Part model, mm, in its own coordinate system. Round coordinates to 2 decimals unless told otherwise and drop trailing zeros. Return JSON: item names as keys, results as strings. Group by question number.
```python
from build123d import *

# Parameters (mm, degrees)
SKETCH1_R           = 2.1
BOSS_EXTRUDE2_DEPTH = 304.8


with BuildPart() as part:
    # Sketch1 → Boss-Extrude2 (new body)
    with BuildSketch(Plane.XY):
        with BuildLine():
            Line((-8.5, 10), (-4.862792737, 10))
            ThreePointArc((-4.862792737, 10), (-4.598292737, 9.947387679), (-4.374060464, 9.797560464))
            Line((-4.374060464, 9.797560464), (-3.3865, 8.81))
            Line((-3.3865, 8.81), (-3.3865, 8.2))
            Line((-3.3865, 8.2), (-5.5, 8.2))
            Line((-5.5, 8.2), (-5.5, 6.561))
            Line((-5.5, 6.561), (-2.8395, 3.9005))
            Line((-2.8395, 3.9005), (-0.1, 3.9005))
            Line((-0.1, 3.9005), (0, 3.8005))
            Line((0, 3.8005), (0.1, 3.9005))
            Line((0.1, 3.9005), (2.8395, 3.9005))
            Line((2.8395, 3.9005), (5.5, 6.561))
            Line((5.5, 6.561), (5.5, 8.2))
            Line((5.5, 8.2), (3.3865, 8.2))
            Line((3.3865, 8.2), (3.3865, 8.81))
            Line((3.3865, 8.81), (4.374060464, 9.797560464))
            ThreePointArc((4.374060464, 9.797560464), (4.598292737, 9.947387679), (4.862792737, 10))
            Line((4.862792737, 10), (8.5, 10))
            ThreePointArc((8.5, 10), (9.560660172, 9.560660172), (10, 8.5))
            Line((10, 8.5), (10, 4.862792737))
            ThreePointArc((10, 4.862792737), (9.947387679, 4.598292737), (9.797560464, 4.374060464))
            Line((9.797560464, 4.374060464), (8.81, 3.3865))
            Line((8.81, 3.3865), (8.2, 3.3865))
            Line((8.2, 3.3865), (8.2, 5.5))
            Line((8.2, 5.5), (6.561, 5.5))
            Line((6.561, 5.5), (3.9005, 2.8395))
            Line((3.9005, 2.8395), (3.9005, 0.1))
            Line((3.9005, 0.1), (3.8005, 0))
            Line((3.8005, 0), (3.9005, -0.1))
            Line((3.9005, -0.1), (3.9005, -2.8395))
            Line((3.9005, -2.8395), (6.561, -5.5))
            Line((6.561, -5.5), (8.2, -5.5))
            Line((8.2, -5.5), (8.2, -3.3865))
            Line((8.2, -3.3865), (8.81, -3.3865))
            Line((8.81, -3.3865), (9.797560464, -4.374060464))
            ThreePointArc((9.797560464, -4.374060464), (9.947387679, -4.598292737), (10, -4.862792737))
            Line((10, -4.862792737), (10, -15.137207263))
            ThreePointArc((10, -15.137207263), (9.947387679, -15.401707263), (9.797560464, -15.625939536))
            Line((9.797560464, -15.625939536), (8.81, -16.6135))
            Line((8.81, -16.6135), (8.2, -16.6135))
            Line((8.2, -16.6135), (8.2, -14.5))
            Line((8.2, -14.5), (6.561, -14.5))
            Line((6.561, -14.5), (3.9005, -17.1605))
            Line((3.9005, -17.1605), (3.9005, -19.9))
            Line((3.9005, -19.9), (3.8005, -20))
            Line((3.8005, -20), (3.9005, -20.1))
            Line((3.9005, -20.1), (3.9005, -22.8395))
            Line((3.9005, -22.8395), (6.561, -25.5))
            Line((6.561, -25.5), (8.2, -25.5))
            Line((8.2, -25.5), (8.2, -23.3865))
            Line((8.2, -23.3865), (8.81, -23.3865))
            Line((8.81, -23.3865), (9.797560464, -24.374060464))
            ThreePointArc((9.797560464, -24.374060464), (9.947387679, -24.598292737), (10, -24.862792737))
            Line((10, -24.862792737), (10, -28.5))
            ThreePointArc((10, -28.5), (9.560660172, -29.560660172), (8.5, -30))
            Line((8.5, -30), (4.862792737, -30))
            ThreePointArc((4.862792737, -30), (4.598292737, -29.947387679), (4.374060464, -29.797560464))
            Line((4.374060464, -29.797560464), (3.3865, -28.81))
            Line((3.3865, -28.81), (3.3865, -28.2))
            Line((3.3865, -28.2), (5.5, -28.2))
            Line((5.5, -28.2), (5.5, -26.561))
            Line((5.5, -26.561), (2.8395, -23.9005))
            Line((2.8395, -23.9005), (0.1, -23.9005))
            Line((0.1, -23.9005), (0, -23.8005))
            Line((0, -23.8005), (-0.1, -23.9005))
            Line((-0.1, -23.9005), (-2.8395, -23.9005))
            Line((-2.8395, -23.9005), (-5.5, -26.561))
            Line((-5.5, -26.561), (-5.5, -28.2))
            Line((-5.5, -28.2), (-3.3865, -28.2))
            Line((-3.3865, -28.2), (-3.3865, -28.81))
            Line((-3.3865, -28.81), (-4.374060464, -29.797560464))
            ThreePointArc((-4.374060464, -29.797560464), (-4.598292737, -29.947387679), (-4.862792737, -30))
            Line((-4.862792737, -30), (-8.5, -30))
            ThreePointArc((-8.5, -30), (-9.560660172, -29.560660172), (-10, -28.5))
            Line((-10, -28.5), (-10, -24.862792737))
            ThreePointArc((-10, -24.862792737), (-9.947387679, -24.598292737), (-9.797560464, -24.374060464))
            Line((-9.797560464, -24.374060464), (-8.81, -23.3865))
            Line((-8.81, -23.3865), (-8.2, -23.3865))
            Line((-8.2, -23.3865), (-8.2, -25.5))
            Line((-8.2, -25.5), (-6.561, -25.5))
            Line((-6.561, -25.5), (-3.9005, -22.8395))
            Line((-3.9005, -22.8395), (-3.9005, -20.1))
            Line((-3.9005, -20.1), (-3.8005, -20))
            Line((-3.8005, -20), (-3.9005, -19.9))
            Line((-3.9005, -19.9), (-3.9005, -17.1605))
            Line((-3.9005, -17.1605), (-6.561, -14.5))
            Line((-6.561, -14.5), (-8.2, -14.5))
            Line((-8.2, -14.5), (-8.2, -16.6135))
            Line((-8.2, -16.6135), (-8.81, -16.6135))
            Line((-8.81, -16.6135), (-9.797560464, -15.625939536))
            ThreePointArc((-9.797560464, -15.625939536), (-9.947387679, -15.401707263), (-10, -15.137207263))
            Line((-10, -15.137207263), (-10, -4.862792737))
            ThreePointArc((-10, -4.862792737), (-9.947387679, -4.598292737), (-9.797560464, -4.374060464))
            Line((-9.797560464, -4.374060464), (-8.81, -3.3865))
            Line((-8.81, -3.3865), (-8.2, -3.3865))
            Line((-8.2, -3.3865), (-8.2, -5.5))
            Line((-8.2, -5.5), (-6.561, -5.5))
            Line((-6.561, -5.5), (-3.9005, -2.8395))
            Line((-3.9005, -2.8395), (-3.9005, -0.1))
            Line((-3.9005, -0.1), (-3.8005, 0))
            Line((-3.8005, 0), (-3.9005, 0.1))
            Line((-3.9005, 0.1), (-3.9005, 2.8395))
            Line((-3.9005, 2.8395), (-6.561, 5.5))
            Line((-6.561, 5.5), (-8.2, 5.5))
            Line((-8.2, 5.5), (-8.2, 3.3865))
            Line((-8.2, 3.3865), (-8.81, 3.3865))
            Line((-8.81, 3.3865), (-9.797560464, 4.374060464))
            ThreePointArc((-9.797560464, 4.374060464), (-9.947387679, 4.598292737), (-10, 4.862792737))
            Line((-10, 4.862792737), (-10, 8.5))
            ThreePointArc((-10, 8.5), (-9.560660172, 9.560660172), (-8.5, 10))
        make_face()
        with Locations(Location((0, 0, 0), (0, 0, 180))):
            Circle(SKETCH1_R, mode=Mode.SUBTRACT)
        with Locations(Location((0, -20, 0), (0, 0, 180))):
            Circle(SKETCH1_R, mode=Mode.SUBTRACT)
        Polygon((-8.2, -12.7), (-8.2, -7.3), (-6.239, -7.3), (-5.5, -6.561), (-2.8395, -3.9005), (-0.1, -3.9005), (0, -3.8005), (0.1, -3.9005), (2.8395, -3.9005), (5.5, -6.561), (6.239, -7.3), (8.2, -7.3), (8.2, -12.7), (6.239, -12.7), (5.5, -13.439), (2.8395, -16.0995), (0.1, -16.0995), (0, -16.1995), (-0.1, -16.0995), (-2.8395, -16.0995), (-5.5, -13.439), (-6.239, -12.7), align=None, mode=Mode.SUBTRACT)
    extrude(amount=BOSS_EXTRUDE2_DEPTH)


solid = part.part
```
Item 1: Flat gauge pins, fed straight in: P1, Ø0.8, axis at y = -2, z = 188.5, coming from the +X side; P2, Ø0.6, axis at x = -4.5, z = 99, coming from the +Y side; P3, Ø1.4, axis at y = -21.5, z = 141.5, coming from the -X side. Where does each tip first touch, or does it go through?
Item 2: Two-plate mould, pull along X, no slides. Class faces 1 (the face through (10, -10, 150)), 2 (the face through (8.2, -10, 150)), 3 (the face through (5, -5, 0)), 4 (the face through (-8.2, -10, 150)): released by +X, released by -X, zero draft, split by the parting line, or undercut.
Item 3: Wall check: L1, parallel to Y at x = -8, z = 250; L2, parallel to Y at x = 0, z = 65.5; L3, parallel to X at y = -20, z = 186. Give the ranges that are in metal, low to high.
Item 4: Cut at A-A (z = 80). State how many separate pieces and enclosed holes the cut face has, then the cut area to 3 significant figures.
Checks:
{
 "1": {"P1": "stops at x = 3.9", "P2": "stops at y = 10", "P3": "stops at x = -3.9"},
 "2": {"face 1": "released by +X", "face 2": "undercut", "face 3": "zero draft", "face 4": "undercut"},
 "3": {"L1": "y = -30 to -25.5, -14.5 to -12.7, -7.3 to -5.5, 5.5 to 10", "L2": "y = -23.8 to -22.1, -17.9 to -16.2, -3.8 to -2.1, 2.1 to 3.8", "L3": "x = -3.8 to -2.1, 2.1 to 3.8"},
 "4": {"separate pieces": "1", "enclosed holes": "3", "area": "297 mm2"}
}
